Drawing for the job (mm, zero at the part's lowest x, y, z). Coordinates: 2 decimals unless noted, no trailing zeros. Write each loop counter-clockwise with the first axis right and the second up, starting at its lowest first coordinate (ties: lowest second). Pieces come first, ordered by that corner, then holes.
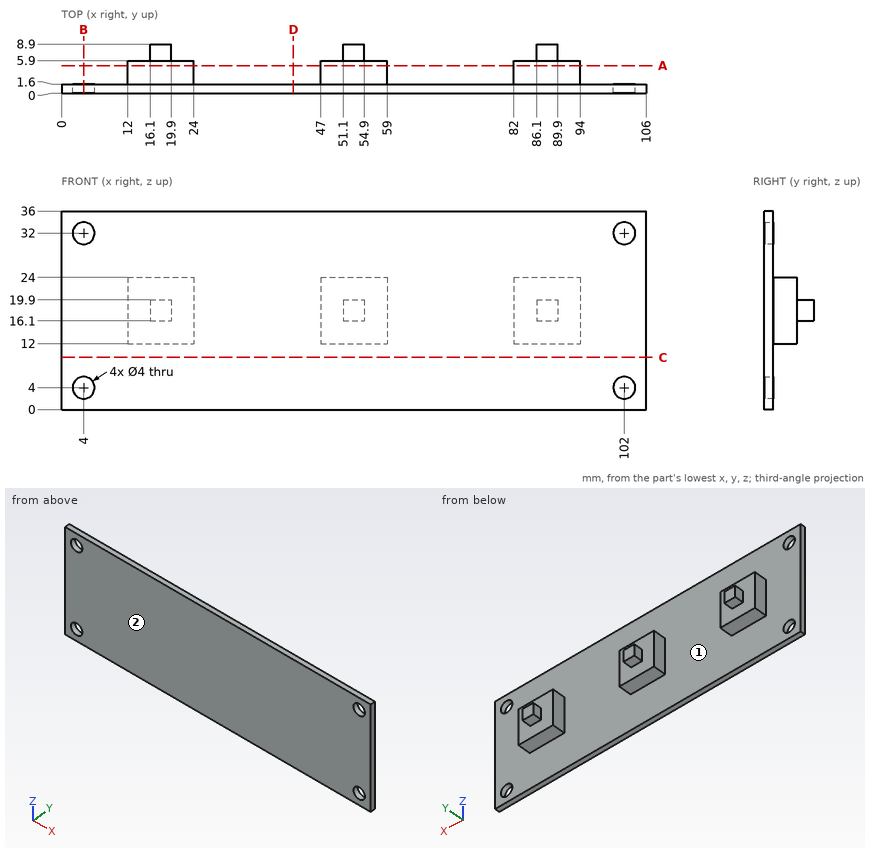
Item 1: Wall check: line 1 along X through (y, z) = (1, 4); line 2 along X through (y, z) = (2.5, 14); line 3 along Y through (x, z) = (87, 32.5). Give the ranges that are in metal, low to high.
Item 2: Two-plate mould, pull along X, no slides. Class the marked faces 1 and 2: +X half, -X half, draft (parallel to the pull), parting line (faces both ways), or undercut.
Item 3: Saw through at A-A, the plane y = 5. Write the cut outline in (x, z).
Item 4: Saw through at B-B, the plane x = 4. Write the cut outline in (y, z), and give its area (3 significant figures).
Item 5: Saw through at D-D, the plane x = 42. Write the cut outline in (y, z).
Item 6: Flat gauge pins, fed straight in: pin 1 Ø4.5 at (x, y) = (20, 4) entering from +Z; pin 2 Ø2.5 at (x, z) = (102, 32) entering from +Y; pin 3 Ø1.5 at (y, z) = (7, 18) entering from -X; pin 4 Ø3 at (x, y) = (11, 5.5) entering from -Z. Where does each tip first touch, or does it go through?
Item 7: Saw through at C-C, the plane z = 9.5. Write the cut outline in (x, y).
Working result:
1. line 1: x = 0 to 2, 6 to 100, 104 to 106
1. line 2: x = 12 to 24, 47 to 59, 82 to 94
1. line 3: y = 0 to 1.6
2. face 1: undercut
2. face 2: draft
3. outline: (12, 12) - (24, 12) - (24, 24) - (12, 24) - close; (47, 12) - (59, 12) - (59, 24) - (47, 24) - close; (82, 12) - (94, 12) - (94, 24) - (82, 24) - close
4. outline: (0, 0) - (1.6, 0) - (1.6, 2) - (0, 2) - close; (0, 6) - (1.6, 6) - (1.6, 30) - (0, 30) - close; (0, 34) - (1.6, 34) - (1.6, 36) - (0, 36) - close
4. area: 44.8 mm2
5. outline: (0, 0) - (1.6, 0) - (1.6, 36) - (0, 36) - close
6. pin 1: stops at z = 24
6. pin 2: passes through
6. pin 3: stops at x = 16.1
6. pin 4: stops at z = 12
7. outline: (0, 0) - (106, 0) - (106, 1.6) - (0, 1.6) - close
